The drawing under review shows one solid part. Ordinate dimensions are in mm from its lowest x, y, z. A direction names the side the tool comes from. Coordinates: 2 decimals unless noted, no trailing zeros. Loops run counter-clockwise (first coordinate to the right, second up) from the corner with the lowest first, then second, coordinate; pieces in that order, holes last. Notation, with made-up numbers: (11.5, -37.75) - (64.5, -37.75) arc R9 cw to (64.5, -22.75) - close; hole circle Ø5 at (88.25, -23). An arc over 180 degrees is marked (long way). Answer as a JSON object with one key per item and string values. Group by question number.
Item 1: Mouldability with a two-part tool opening along X and no side actions: class the marked faces 1, 2 and 3 as released by +X, released by -X, zero draft, split by the parting line, or undercut.
Item 2: We need section D-D (y = 1.5). Give the boundary of the cut face in (x, z).
Item 3: We need section B-B (x = 20). Give the boundary of the cut face in (y, z), then the cut area to 3 significant figures.
Item 4: Clearance check with flat-ended pins moving along their axes: pin 1 (13.5 mm diameter, centred on x = 27, z = 12.5, fed in from +Y); pin 2 (1.5 mm diameter, centred on y = 6.5, z = 21, fed in from +X); pin 3 (2 mm diameter, centred on y = 2, z = 4.5, fed in from +X); pin 4 (11.5 mm diameter, centred on x = 20, z = 18, fed in from +Y). State where each tip first meets the part, or that it passes through.
Item 5: Tool access review of the marked faces 4 and 5: name each direction out of +Z, -Z, +X, -X, +Y, -Y from which nothing blocks a thin tool from reaching the whole face with its end or side.
Item 6: We need section C-C (z = 23.25). Give the boundary of the cut face in (x, y).
Item 7: To check wall thickness, follow line 1 (X direction, y = 3.4, z = 18); line 2 (Z direction, x = 40.5, y = 8); line 3 (Z direction, x = 40, y = 1.75). State the ranges of each line that lie inside material, in increasing order.
Item 8: We need section A-A (y = 8). Give the boundary of the cut face in (x, z).
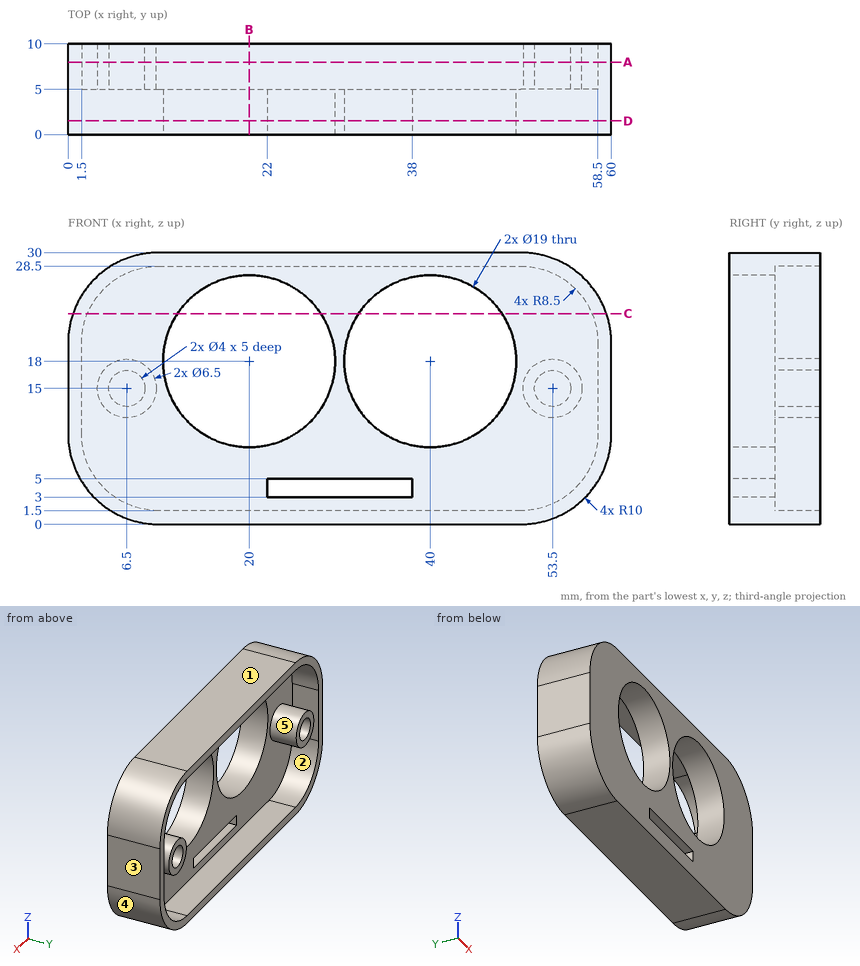
Check sheet entries:
{
 "1": {"face 1": "zero draft", "face 2": "undercut", "face 3": "released by +X"},
 "2": {"outline": "(0, 10) arc R10 ccw to (10, 0) - (50, 0) arc R10 ccw to (60, 10) - (60, 20) arc R10 ccw to (50, 30) - (10, 30) arc R10 ccw to (0, 20) - close; hole circle Ø19 at (20, 18); hole (22, 3) - (38, 3) - (38, 5) - (22, 5) - close; hole circle Ø19 at (40, 18)"},
 "3": {"outline": "(0, 0) - (10, 0) - (10, 1.5) - (5, 1.5) - (5, 8.5) - (0, 8.5) - close; (0, 27.5) - (5, 27.5) - (5, 28.5) - (10, 28.5) - (10, 30) - (0, 30) - close", "area": "70.0 mm2"},
 "4": {"pin 1": "stops at y = 5", "pin 2": "stops at x = 60", "pin 3": "stops at x = 58.93", "pin 4": "passes through"},
 "5": {"face 4": "-Z, +X, +Y, -Y", "face 5": "+Y"},
 "6": {"outline": "(0.54, 0) - (12.08, 0) - (12.08, 5) - (2.15, 5) - (2.15, 10) - (0.54, 10) - close; (27.92, 0) - (32.08, 0) - (32.08, 5) - (27.92, 5) - close; (47.92, 0) - (59.46, 0) - (59.46, 10) - (57.85, 10) - (57.85, 5) - (47.92, 5) - close"},
 "7": {"line 1": "x = 0 to 10.5, 29.5 to 30.5, 49.5 to 60", "line 2": "z = 0 to 1.5, 28.5 to 30", "line 3": "z = 0 to 8.5, 27.5 to 30"},
 "8": {"outline": "(0, 10) arc R10 ccw to (10, 0) - (50, 0) arc R10 ccw to (60, 10) - (60, 20) arc R10 ccw to (50, 30) - (10, 30) arc R10 ccw to (0, 20) - close; circle Ø6.5 at (6.5, 15); circle Ø6.5 at (53.5, 15); hole (1.5, 10) arc R8.5 ccw to (10, 1.5) - (50, 1.5) arc R8.5 ccw to (58.5, 10) - (58.5, 20) arc R8.5 ccw to (50, 28.5) - (10, 28.5) arc R8.5 ccw to (1.5, 20) - close; hole circle Ø4 at (6.5, 15); hole circle Ø4 at (53.5, 15)"}
}
